from build123d import *

# Parameters (mm, degrees)
SKETCH1_W           = 130
SKETCH1_H           = 130
BOSS_EXTRUDE1_DEPTH = 5
FILLET1_R           = 20
CHAMFER1_SIZE       = 20


with BuildPart() as part:
    # Sketch1 → Boss-Extrude1 (new body)
    with BuildSketch(Plane.XY):
        with Locations((65, 65)):
            Rectangle(SKETCH1_W, SKETCH1_H)
    extrude(amount=BOSS_EXTRUDE1_DEPTH)

    # Fillet1
    fillet1_edges = [part.edges().sort_by_distance(p)[0] for p in [
        (130, 0, 2.5),
    ]]
    fillet(fillet1_edges, radius=FILLET1_R)

    # Chamfer1
    chamfer1_edges = [part.edges().sort_by_distance(p)[0] for p in [
        (0, 130, 2.5),
    ]]
    chamfer(chamfer1_edges, length=CHAMFER1_SIZE)


solid = part.part
The listing builds one solid part. Answer for the finished solid, in the listing's coordinates (mm). Round coordinates to 2 decimals unless told otherwise and drop trailing zeros. Write each loop counter-clockwise with the first axis right and the second up, starting at its lowest first coordinate (ties: lowest second). Pieces come first, ordered by that corner, then holes. Notation, with made-up numbers: M 3.25,1 L 20.25,1 A23 ccw 20.25,12 Z; hole C -22,41 d6. An arc over 180 degrees is marked long. Write each question's results on one line, items separated by ' | '. Start each with the question number.
Item 1: A cutting plane is placed at A-A on z = 2.2. Write down the section's boundary in (x, y).
Item 2: For a pull along Z with two mould halves and no side action, classify faces 1 (the face through (64, 66, 0)), 2 (the face through (0, 54, 2)), 3 (the face through (64, 66, 5)) as pulls with the +Z half, pulls with the -Z half, needs draft (parallel to the pull), parting line crosses it, or undercut.
Item 3: A cutting plane is placed at B-B on x = 9. Write down the section's boundary in (y, z), and give its area (3 significant figures).
Item 4: Flat-ended cylindrical pins translate along their axes: pin 1 Ø2 at (x, z) = (117, 1.5) entering from -Y; pin 2 Ø3 at (x, z) = (115, 1) entering from -Y. Find the tip coordinate at first contact, or state that the pin passes through.
Item 5: Straight lines are drawn through the part: L1, parallel to X at y = 19.5, z = 1.7; L2, parallel to X at y = 7, z = 3.75; L3, parallel to Y at x = 115, z = 3.95. For each, find the intervals that lie inside material, in ascending order. Write a range as [from, to].
Item 6: A cutting plane is placed at C-C on x = 122.5. Write down the section's boundary in (y, z).
Check sheet entries:
1) outline: M 0,0 L 110,0 A20 ccw 130,20 L 130,130 L 20,130 L 0,110 Z
2) face 1: pulls with the -Z half | face 2: needs draft | face 3: pulls with the +Z half
3) outline: M 0,0 L 119,0 L 119,5 L 0,5 Z | area: 595 mm²
4) pin 1: y = 0.92 | pin 2: y = 0.31
5) L1: [0, 129.99] | L2: [0, 125.2] | L3: [0.64, 130]
6) outline: M 4.39,0 L 130,0 L 130,5 L 4.39,5 Z
